Design review of the part shown in the three views and the two pictorial views. Dimensions are in mm from the part's minimum x, y and z. Coordinates: 2 decimals unless noted, no trailing zeros. Write each loop counter-clockwise with the first axis right and the second up, starting at its lowest first coordinate (ties: lowest second). Pieces come first, ordered by that corner, then holes. Notation, with made-up numbers: (-21.75, 65.5) - (22.25, 65.5) arc R21 ccw to (22.25, 96.5) - close; hole circle Ø11 at (-13, -17). An arc over 180 degrees is marked (long way). Return JSON: item names as keys, results as strings. Group by question number.
(1) We need section A-A on y = 25. State the section outline as (x, z) points (3 decimals), then the cut area to 3 significant figures.
(2) We need section C-C on z = 1.1. State the section outline as (x, y) points (3 decimals), then the cut area to 3 significant figures.
(3) We need section B-B on x = 25. State the section outline as (y, z) points (3 decimals).
(4) We need section D-D on y = 30.5. State the section outline as (x, z) points (3 decimals), then the cut area to 3 significant figures.
(5) To check wall thickness, follow L1, parallel to Y at x = 25, z = 1.3 (3 decimals). State the ranges of the line that lie inside material, in increasing order. Write a range as from..to.
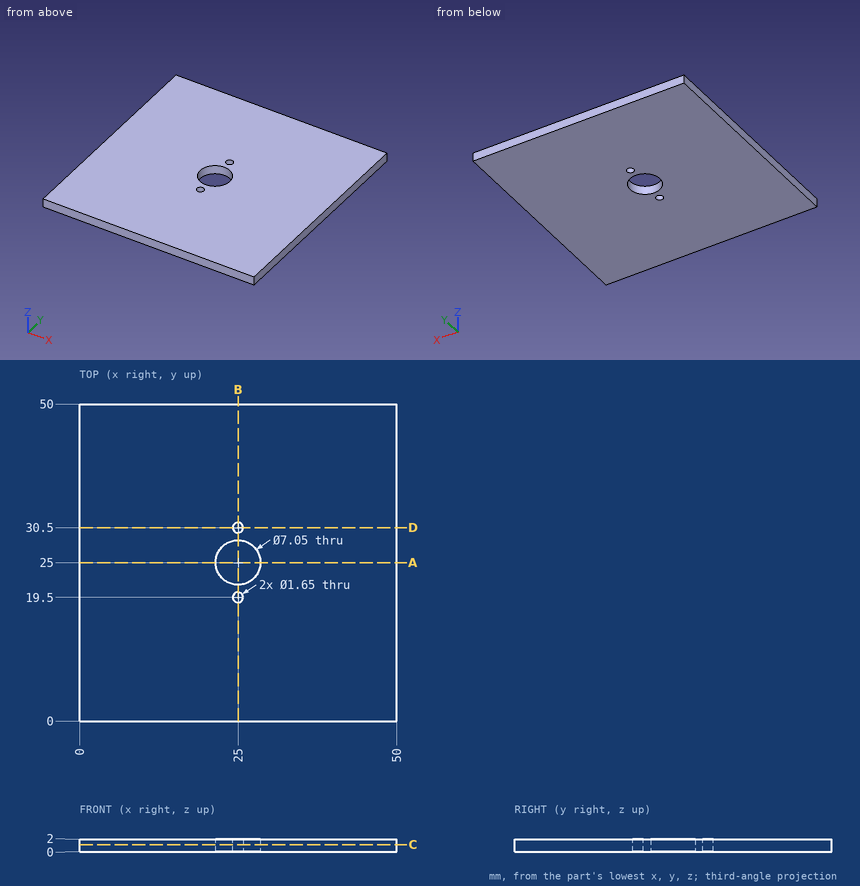
Ans:
{
 "1": {"outline": "(0, 0) - (21.475, 0) - (21.475, 2) - (0, 2) - close; (28.525, 0) - (50, 0) - (50, 2) - (28.525, 2) - close", "area": "85.9 mm²"},
 "2": {"outline": "(0, 0) - (50, 0) - (50, 50) - (0, 50) - close; hole circle Ø7.05 at (25, 25); hole circle Ø1.65 at (25, 19.5); hole circle Ø1.65 at (25, 30.5)", "area": "2,460 mm²"},
 "3": {"outline": "(0, 0) - (18.675, 0) - (18.675, 2) - (0, 2) - close; (20.325, 0) - (21.475, 0) - (21.475, 2) - (20.325, 2) - close; (28.525, 0) - (29.675, 0) - (29.675, 2) - (28.525, 2) - close; (31.325, 0) - (50, 0) - (50, 2) - (31.325, 2) - close"},
 "4": {"outline": "(0, 0) - (24.175, 0) - (24.175, 2) - (0, 2) - close; (25.825, 0) - (50, 0) - (50, 2) - (25.825, 2) - close", "area": "96.7 mm²"},
 "5": {"L1": "0..18.675, 20.325..21.475, 28.525..29.675, 31.325..50"}
}
